```python
from build123d import *

# Parameters (mm, degrees)
BOSS_EXTRUDE1_DEPTH     = 50.8
CUT_EXTRUDE1_DEPTH      = 25.4
CUT_EXTRUDE2_START      = -102.6
SKETCH3_R               = 12.7
CUT_EXTRUDE2_DEPTH      = 103.6
SKETCH4_R               = 19.05
CUT_EXTRUDE3_DEPTH      = 1
CUT_EXTRUDE3_DEPTH_BACK = 458.2
FILLET1_R               = 16.51


with BuildPart() as part:
    # Sketch1 → Boss-Extrude1 (new body, symmetric)
    with BuildSketch(Plane(origin=(0, 0, 0), x_dir=(1, 0, 0), z_dir=(0, 1, 0))):
        with BuildLine():
            Line((76.2, -25.4), (-76.2, -25.4))
            Line((-76.2, -25.4), (-76.2, -152.4))
            ThreePointArc((-76.2, -152.4), (-98.518463274, -206.281536726), (-152.4, -228.6))
            Line((-152.4, -228.6), (-482.6, -228.6))
            Line((-482.6, -228.6), (-482.6, 228.6))
            Line((-482.6, 228.6), (-152.4, 228.6))
            ThreePointArc((-152.4, 228.6), (-98.518463274, 206.281536726), (-76.2, 152.4))
            Line((-76.2, 152.4), (-76.2, 25.4))
            Line((-76.2, 25.4), (76.2, 25.4))
            Line((76.2, 25.4), (76.2, 63.5))
            ThreePointArc((76.2, 63.5), (79.919743879, 72.480256121), (88.9, 76.2))
            Line((88.9, 76.2), (114.3, 76.2))
            ThreePointArc((114.3, 76.2), (123.280256121, 72.480256121), (127, 63.5))
            Line((127, 63.5), (127, -63.5))
            ThreePointArc((127, -63.5), (123.280256121, -72.480256121), (114.3, -76.2))
            Line((114.3, -76.2), (88.9, -76.2))
            ThreePointArc((88.9, -76.2), (79.919743879, -72.480256121), (76.2, -63.5))
            Line((76.2, -63.5), (76.2, -25.4))
        make_face()
    extrude(amount=BOSS_EXTRUDE1_DEPTH, both=True)

    # Sketch2 → Cut-Extrude1 (cut, symmetric)
    with BuildSketch(Plane(origin=(0, 0, 0), x_dir=(1, 0, 0), z_dir=(0, 1, 0))):
        with BuildLine():
            Line((127, -63.5), (127, -25.4))
            Line((127, -25.4), (76.2, -25.4))
            Line((76.2, -25.4), (76.2, -63.5))
            ThreePointArc((76.2, -63.5), (79.919743879, -72.480256121), (88.9, -76.2))
            Line((88.9, -76.2), (114.3, -76.2))
            ThreePointArc((114.3, -76.2), (123.280256121, -72.480256121), (127, -63.5))
        make_face()
    cut_extrude1 = extrude(amount=CUT_EXTRUDE1_DEPTH, both=True, mode=Mode.SUBTRACT)

    # Sketch3 → Cut-Extrude2 (cut)
    with BuildSketch(Plane(origin=(0, 50.8, 0), x_dir=(1, 0, 0), z_dir=(0, 1, 0)).offset(CUT_EXTRUDE2_START)):
        with Locations((101.6, -50.8)):
            Circle(SKETCH3_R)
    cut_extrude2 = extrude(amount=CUT_EXTRUDE2_DEPTH, mode=Mode.SUBTRACT)

    # Mirror1: Cut-Extrude1, Cut-Extrude2 across plane
    add(cut_extrude1.mirror(Plane.XY), mode=Mode.SUBTRACT)
    add(cut_extrude2.mirror(Plane.XY), mode=Mode.SUBTRACT)

    # Sketch4 → Cut-Extrude3 (cut, two sides)
    with BuildSketch(Plane.XY.offset(228.6)) as cut_extrude3_sk:
        with Locations((-406.4, 0)):
            Circle(SKETCH4_R)
    extrude(amount=CUT_EXTRUDE3_DEPTH, mode=Mode.SUBTRACT)
    extrude(cut_extrude3_sk.sketch, amount=-CUT_EXTRUDE3_DEPTH_BACK, mode=Mode.SUBTRACT)

    # Fillet1
    fillet1_edges = [part.edges().sort_by_distance(p)[0] for p in [
        (-482.6, 0, -228.6),
        (-76.2, 0, -25.4),
        (-482.6, 0, 228.6),
    ]]
    fillet(fillet1_edges, radius=FILLET1_R)


solid = part.part
```
Geometry check sheet. Reference: the model listing, model coordinates, mm. A direction names the side the tool comes from. Coordinates: 2 decimals unless noted, no trailing zeros. Write each loop counter-clockwise with the first axis right and the second up, starting at its lowest first coordinate (ties: lowest second). Pieces come first, ordered by that corner, then holes. Notation, with made-up numbers: M 0.25,72 L 42.25,72 A13 ccw 42.25,76 Z; hole C 73.25,45 d2. An arc over 180 degrees is marked long. One line per item, written item: value. Start each with the question number.
(1) Sectioned sample at B-B, the plane z = 50.8. Enter the section's corners in (x, y), and give its area (3 significant figures).
(2) Sectioned sample at A-A, the plane x = -406.4. Enter the section's corners in (y, z), and give its area (3 significant figures).
(3) Tool access check on faces 4 (the face through (-76.2, 1, -98)), 5 (the face through (96, -25.4, 39)), 6 (the face through (96, 25.4, -39)), 7 (the face through (80.02, 38.28, 72.58)), 8 (the face through (-477.89, -0.71, -223.64)). Record the directions out of +Z, -Z, +X, -X, +Y, -Y that give a thin tool (end or side, any length) a straight path to the whole face; none if there is none.
(4) Release check for a two-part mould opening along Y. For faces 1 (the face through (-99.114, 0.711, -206.871)), 2 (the face through (32, 1, -25.4)), 3 (the face through (27, 1, 25.4)) record: released by +Y, released by -Y, zero draft, split by the parting line, or undercut.
(5) Scan lines: line 1 along Z through (x, y) = (101.6, -37.25); line 2 along X through (y, z) = (34, -50); line 3 along Y through (x, z) = (-406.4, 107.5). Record each from-to range of solid material in increasing order. Write a range as [from, to].
(6) Depth check by flat-ended pin: pin 1 (7.5 mm diameter, centred on x = 99, y = -44.5, fed in from +Z); pin 2 (5 mm diameter, centred on x = -149.5, y = -23.5, fed in from -Z); pin 3 (23 mm diameter, centred on x = 101.6, z = 50.8, fed in from +Y); pin 4 (1 mm diameter, centred on x = -87, y = -34.5, fed in from +Z). Enter the tip coordinate at first touch or a pass-through.
(7) Sectioned sample at D-D, the plane x = 101.6. Enter the section's corners in (y, z).
(8) Sectioned sample at C-C, the plane y = 39.5. Enter the section's corners in (x, z).
Filled sheet:
1. outline: M -482.6,-50.8 L -76.2,-50.8 L -76.2,50.8 L -482.6,50.8 Z; M 76.2,-50.8 L 88.9,-50.8 L 88.9,-25.4 L 76.2,-25.4 Z; M 76.2,25.4 L 88.9,25.4 L 88.9,50.8 L 76.2,50.8 Z; M 114.3,-50.8 L 127,-50.8 L 127,-25.4 L 114.3,-25.4 Z; M 114.3,25.4 L 127,25.4 L 127,50.8 L 114.3,50.8 Z; hole C -406.4,0 d38.1
1. area: 41,400 mm²
2. outline: M -50.8,-228.6 L -19.05,-228.6 L -19.05,228.6 L -50.8,228.6 Z; M 19.05,-228.6 L 50.8,-228.6 L 50.8,228.6 L 19.05,228.6 Z
2. area: 29,000 mm²
3. face 4: -Z, +Y, -Y
3. face 5: +Z, +X
3. face 6: -Z, +X
3. face 7: +Z, +Y, -Y
3. face 8: -Z, -X, +Y, -Y
4. face 1: zero draft
4. face 2: undercut
4. face 3: undercut
5. line 1: [-76.2, -63.5], [-38.1, 38.1], [63.5, 76.2]
5. line 2: [-482.6, -76.2], [76.2, 88.93], [114.27, 127]
5. line 3: [-50.8, -19.05], [19.05, 50.8]
6. pin 1: z = 76.2
6. pin 2: z = -228.6
6. pin 3: through
6. pin 4: z = 192.33
7. outline: M -50.8,-76.2 L -25.4,-76.2 L -25.4,-63.5 L -50.8,-63.5 Z; M -50.8,-38.1 L -25.4,-38.1 L -25.4,-25.4 L 25.4,-25.4 L 25.4,-38.1 L 50.8,-38.1 L 50.8,38.1 L 25.4,38.1 L 25.4,25.4 L -25.4,25.4 L -25.4,38.1 L -50.8,38.1 Z; M -50.8,63.5 L -25.4,63.5 L -25.4,76.2 L -50.8,76.2 Z; M 25.4,-76.2 L 50.8,-76.2 L 50.8,-63.5 L 25.4,-63.5 Z; M 25.4,63.5 L 50.8,63.5 L 50.8,76.2 L 25.4,76.2 Z
8. outline: M -482.6,-212.09 A16.51 ccw -466.09,-228.6 L -152.4,-228.6 A76.2 ccw -76.2,-152.4 L -76.2,-41.91 A16.51 cw -59.69,-25.4 L 76.2,-25.4 L 76.2,-63.5 A12.7 ccw 88.9,-76.2 L 114.3,-76.2 A12.7 ccw 127,-63.5 L 127,63.5 A12.7 ccw 114.3,76.2 L 88.9,76.2 A12.7 ccw 76.2,63.5 L 76.2,25.4 L -76.2,25.4 L -76.2,152.4 A76.2 ccw -152.4,228.6 L -466.09,228.6 A16.51 ccw -482.6,212.09 Z; hole C 101.6,-50.8 d25.4; hole C 101.6,50.8 d25.4
